Geometry check sheet. Reference: the model listing, model coordinates, mm. A direction names the side the tool comes from. Coordinates: 2 decimals unless noted, no trailing zeros. Write each loop counter-clockwise with the first axis right and the second up, starting at its lowest first coordinate (ties: lowest second). Pieces come first, ordered by that corner, then holes. Notation, with made-up numbers: M 23.25,65 L 40.25,65 A11 cw 40.25,78 Z; hole C -20.75,27 d9. An arc over 180 degrees is marked long. Write each question's results on one line, items separated by ' | '.
```python
from build123d import *

# Parameters (mm, degrees)
F0_R     = 57.15
F1_DEPTH = 101.092
F2_SIZE  = 57.15
F3_T     = -2.54


with BuildPart() as f1:
    # F0 (on Front) → F1 (new body)
    with BuildSketch(Plane.XZ):
        Circle(F0_R)
    extrude(amount=F1_DEPTH)

    # F2
    f2_edges = [f1.edges().sort_by_distance(p)[0] for p in [
        (-57.15, -101.092, 0),
    ]]
    chamfer(f2_edges, length=F2_SIZE)

    # F3
    f3_openings = [f1.faces().sort_by_distance(p)[0] for p in [
        (0, 0, 0),
    ]]
    offset(amount=F3_T, openings=f3_openings)


solid = f1.part
```
Q1. Sectioned sample at B-B on y = -83. Record the cut outline in (x, z), and give its area (3 significant figures).
Geometry check:
outline: C 0,0 d36.18; hole C 0,0 d29 | area: 368 mm2
Q2. Sectioned sample at A-A on y = -34.5. Record the cut outline in (x, z).
Geometry check:
outline: C 0,0 d114.3; hole C 0,0 d109.22
Q3. Access from +Z, -Z, +X, -X, +Y, -Y to the whole of each face (thin tool, end or side, straight path). Record for faces 4 (the cylindrical face through (-57.095, -21.663, 2.513)), 5 (the cylindrical face through (-7.109, -21.145, 54.145)).
Geometry check:
face 4: +Y, -Y | face 5: +Y
Q4. Mould release check, pull along Z, two halves, no side actions. Record for faces 1 (the conical face through (-3.21, -82.71, -14.44)), 2 (the flat face through (46.3, 0, -29.4)), 3 (the conical face through (14.29, -85.62, -5.93)): pulls with the +Z half, pulls with the -Z half, needs draft (parallel to the pull), parting line crosses it, or undercut.
Geometry check:
face 1: undercut | face 2: needs draft | face 3: parting line crosses it
Q5. Depth check by flat-ended pin: P1, Ø1.5, axis at y = -25, z = -5, coming from the +X side; P2, Ø6, axis at y = -70, z = 36, coming from the -X side; P3, Ø4, axis at x = -4, z = -32, coming from the +Y side; P4, Ø3, axis at x = -34, z = 30, coming from the +Y side. Enter the tip coordinate at first touch or a pass-through.
Geometry check:
P1: stops at x = 56.99 | P2: passes through | P3: stops at y = -63.25 | P4: stops at y = -50.66
Q6. Scan lines: probe 1 along Z at (x, y) = (0, -13); probe 2 along X at (y, z) = (-34, -1); probe 3 along X at (y, z) = (-45, -32). Record each from-to range of solid material in increasing order.
Geometry check:
probe 1: z = -57.15 to -54.61, 54.61 to 57.15 | probe 2: x = -57.14 to -54.6, 54.6 to 57.14 | probe 3: x = -46.07 to -41.62, 41.62 to 46.07
